from build123d import *

# Parameters (mm, degrees)
F0_W     = 254
F0_H     = 203.2
F1_DEPTH = 50.8
F1_TAPER = 20
F2_W     = 152.4
F2_H     = 127
F3_DEPTH = 25.4
F3_TAPER = 20
F4_R     = 10.16
F5_R     = 43.275006419
F6_DEPTH = 146.812


with BuildPart() as f1:
    # F0 (on Top) → F1 (new body)
    with BuildSketch(Plane.XY):
        with Locations((2.1702556405, 0)):
            Rectangle(F0_W, F0_H)
    extrude(amount=F1_DEPTH, taper=F1_TAPER)

    # F2 (on face) → F3 (cut)
    with BuildSketch(Plane.XY.offset(50.8)):
        Rectangle(F2_W, F2_H)
    extrude(amount=-F3_DEPTH, taper=F3_TAPER, mode=Mode.SUBTRACT)

    # F4
    f4_edges = [f1.edges().sort_by_distance(p)[0] for p in [
        (-106.340056, 0, 50.8),
        (2.170256, 83.110312, 50.8),
        (2.170256, -83.110312, 50.8),
        (110.680568, 0, 50.8),
        (76.2, 0, 50.8),
        (0, 63.5, 50.8),
        (-76.2, 0, 50.8),
        (0, -63.5, 50.8),
        (119.925412, -92.355156, 25.4),
        (119.925412, 92.355156, 25.4),
        (-115.5849, -92.355156, 25.4),
        (-115.5849, 92.355156, 25.4),
    ]]
    fillet(f4_edges, radius=F4_R)

    # F5 (on face) → F6 (join)
    with BuildSketch(Plane.XY.offset(25.4)):
        Circle(F5_R)
    extrude(amount=F6_DEPTH)


solid = f1.part
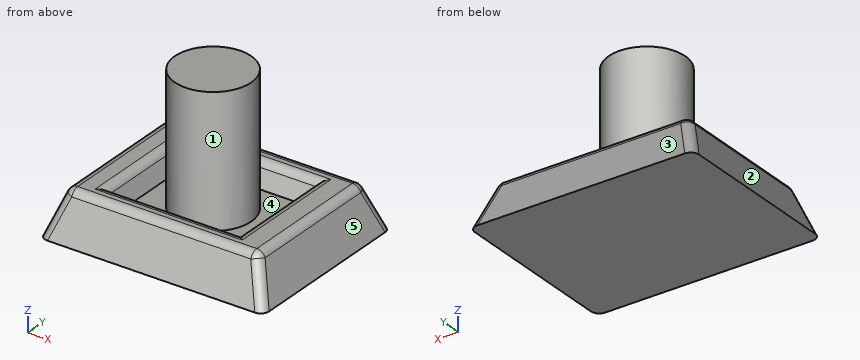
Read the model definition and answer for the solid it produces. Units are mm, in the model's axes. Face numbers are marked on the shaded views. A direction names the side the tool comes from. Round coordinates to 2 decimals unless told otherwise and drop trailing zeros. Loops run counter-clockwise (first coordinate to the right, second up) from the corner with the lowest first, then second, coordinate; pieces in that order, holes last.
Q1. Which of the six approach directions +Z, -Z, +X, -X, +Y, -Y give full straight-line access (tool end or side, diameter ignored) to the marked faces 1 and 2?
Q2. Each of these flat-tipped pins is pushed along its axis until it touches: pin 1 (5 mm diameter, centred on x = -22, z = 147.5, fed in from -Y); pin 2 (3 mm diameter, centred on x = 44.5, y = 37.5, fed in from +Z); pin 3 (3 mm diameter, centred on x = 29.5, z = 144, fed in from +Y). Where does it stop, or does it pass through?
Q3. Determine the mould class of the marked faces 3, 4 and 5 for opening direction Y: released by +Y, released by -Y, zero draft, split by the parting line, or undercut.
Q4. Consider probe 1 along Y at (x, z) = (28, 42.5); probe 2 along X at (y, z) = (2.5, 38); probe 3 along Z at (x, y) = (-3.5, -74). Determine where each line is inside the solid, lowest interval first.
Q5. Section A-A on z = 61 is taken. Write down the section's boundary in (x, y) (3 decimals).
Output:
1. face 1: +Z
1. face 2: +Z, -X, +Y, -Y
2. pin 1: stops at y = -38.63
2. pin 2: stops at z = 25.4
2. pin 3: stops at y = 33
3. face 3: released by +Y
3. face 4: undercut
3. face 5: zero draft
4. probe 1: y = -86.13 to -60.48, -33 to 33, 60.48 to 86.13
4. probe 2: x = -111 to -71.54, -43.2 to 43.2, 71.54 to 115.34
4. probe 3: z = 0 to 50.8
5. outline: circle Ø86.55 at (0, 0)
